Input: part model. Units: mm. Frame: model coordinates. A direction names the side the tool comes from. Coordinates: 2 decimals unless noted, no trailing zeros. Loops run counter-clockwise (first coordinate to the right, second up) from the corner with the lowest first, then second, coordinate; pieces in that order, holes last. Notation, with made-up numbers: (48.25, 72) - (74.25, 72) arc R19 ccw to (74.25, 85) - close; hole circle Ø2 at (-36.75, 76). An arc over 180 degrees is marked (long way). Write item = value, one per line. Start each with the question number.
from build123d import *

# Parameters (mm, degrees)
BOSS_EXTRUDE1_DEPTH   = 4.064
BOSS_EXTRUDE1_2_DEPTH = 4.064
SKETCH1_3_W           = 60.96
SKETCH1_3_H           = 9.652
SKETCH1_3_H_2         = 1.778
BOSS_EXTRUDE2_DEPTH   = 1.524
SKETCH1_6_W           = 60.96
SKETCH1_6_H           = 1.778
BOSS_EXTRUDE3_DEPTH   = 24.13
BOSS_EXTRUDE4_DEPTH   = 38.1
BOSS_EXTRUDE7_DEPTH   = 60.96
BOSS_EXTRUDE8_DEPTH   = 60.96
CUT_EXTRUDE2_START    = -5.08
CUT_EXTRUDE2_DEPTH    = 50.8
SKETCH6_R             = 2.54
CUT_EXTRUDE3_DEPTH    = 89.450736232
BOSS_EXTRUDE9_START   = -27.94
BOSS_EXTRUDE9_DEPTH   = 5.08
BOSS_EXTRUDE10_REACH  = 83.27
CUT_EXTRUDE4_START    = -1.778
CUT_EXTRUDE4_DEPTH    = 57.404


with BuildPart() as part:
    # Sketch1 → Boss-Extrude1 (new body)
    with BuildSketch(Plane(origin=(0, 0, 0), x_dir=(0, 0, -1), z_dir=(1, 0, 0))):
        Polygon((7.62, 0), (0, 0), (0, -11.43), (7.62, -11.43), (7.62, -1.778), align=None)
    extrude(amount=BOSS_EXTRUDE1_DEPTH)



with BuildPart() as body_2:
    # Sketch1 → Boss-Extrude1 2 (new body)
    with BuildSketch(Plane(origin=(0, 0, 0), x_dir=(0, 0, -1), z_dir=(1, 0, 0))):
        Polygon((76.2, 0), (68.58, 0), (68.58, -1.778), (68.58, -11.43), (76.2, -11.43), align=None)
    extrude(amount=BOSS_EXTRUDE1_2_DEPTH)


with BuildPart() as part_1:
    add(part.part)

    add(body_2.part)  # Boss-Extrude2 merges body 2
    # Sketch1<3> → Boss-Extrude2 (add)
    with BuildSketch(Plane(origin=(0, 0, 0), x_dir=(0, 0, -1), z_dir=(1, 0, 0))):
        with Locations((38.1, -6.604)):
            Rectangle(SKETCH1_3_W, SKETCH1_3_H)
        with Locations((38.1, -0.889)):
            Rectangle(SKETCH1_3_W, SKETCH1_3_H_2)
    extrude(amount=BOSS_EXTRUDE2_DEPTH)

    # Sketch1<6> → Boss-Extrude3 (add)
    with BuildSketch(Plane(origin=(0, 0, 0), x_dir=(0, 0, -1), z_dir=(1, 0, 0))):
        with Locations((38.1, -0.889)):
            Rectangle(SKETCH1_6_W, SKETCH1_6_H)
    extrude(amount=-BOSS_EXTRUDE3_DEPTH)

    # Sketch4 → Boss-Extrude4 (add)
    with BuildSketch(Plane.XZ.offset(1.778)):
        Polygon((0, -7.62), (-24.13, -7.62), (-24.13, -68.58), (0, -68.58), (0, -66.802), (-22.352, -66.802), (-22.352, -9.398), (0, -9.398), align=None)
    extrude(amount=-BOSS_EXTRUDE4_DEPTH)

    # Sketch5<4> → Boss-Extrude7 (add)
    with BuildSketch(Plane(origin=(0, 0, -68.58), x_dir=(-1, 0, 0), z_dir=(0, 0, -1))):
        Polygon((1.778, -1.778), (0, -1.778), (0, -3.556), align=None)
    extrude(amount=-BOSS_EXTRUDE7_DEPTH)

    # Sketch5<5> → Boss-Extrude8 (add)
    with BuildSketch(Plane(origin=(0, 0, -68.58), x_dir=(-1, 0, 0), z_dir=(0, 0, -1))):
        Polygon((9.652, -1.778), (5.842, -1.778), (0, -7.62), (0, -11.43), align=None)
    extrude(amount=-BOSS_EXTRUDE8_DEPTH)

    # Sketch5 → Cut-Extrude2 (cut)
    with BuildSketch(Plane(origin=(0, 0, -68.58), x_dir=(-1, 0, 0), z_dir=(0, 0, -1)).offset(CUT_EXTRUDE2_START)):
        Polygon((9.652, -1.778), (5.842, -1.778), (0, -7.62), (0, -11.43), align=None)
    extrude(amount=-CUT_EXTRUDE2_DEPTH, mode=Mode.SUBTRACT)

    # Sketch6 → Cut-Extrude3 (cut, through all)
    with BuildSketch(Plane(origin=(-22.352, 0, 0), x_dir=(0, 0, -1), z_dir=(1, 0, 0))):
        with Locations((23.114, 29.21)):
            Circle(SKETCH6_R)
        with Locations((53.086, 29.21)):
            Circle(SKETCH6_R)
        Polygon((38.1, 20.32), (12.7, 20.32), (12.7, 8.89), (63.5, 8.89), (63.5, 20.32), align=None)
    extrude(amount=-CUT_EXTRUDE3_DEPTH, mode=Mode.SUBTRACT)

    # Sketch5<12> → Boss-Extrude9 (add)
    with BuildSketch(Plane(origin=(0, 0, -68.58), x_dir=(-1, 0, 0), z_dir=(0, 0, -1)).offset(BOSS_EXTRUDE9_START)):
        Polygon((9.652, -1.778), (5.842, -1.778), (0, -7.62), (0, -11.43), align=None)
    extrude(amount=-BOSS_EXTRUDE9_DEPTH)

    # Boss-Extrude10: up to this face of the body (flat: up to its plane)
    boss_extrude10_end = Plane(part_1.part.faces().sort_by_distance((-11.79395977, 16.525022989, -68.58))[0])
    # Sketch9 → Boss-Extrude10 (add, up to the picked face)
    with BuildSketch(Plane.XY.offset(-7.62), mode=Mode.PRIVATE) as boss_extrude10_sk1:
        Polygon((0, 27.94), (0, 30.988), (4.572, 30.988), (4.572, 33.02), (7.140253406, 30.988), (7.140253406, 27.94), align=None)
    boss_extrude10_tool1 = split(extrude(boss_extrude10_sk1.sketch, amount=-BOSS_EXTRUDE10_REACH, mode=Mode.PRIVATE), bisect_by=boss_extrude10_end, keep=Keep.BOTH, mode=Mode.PRIVATE)
    add(boss_extrude10_tool1.solids().sort_by(Axis((3.769039, 29.699674, -7.62), (0, 0, -1)))[0])

    # Sketch9<2> → Cut-Extrude4 (cut)
    with BuildSketch(Plane.XY.offset(-7.62).offset(CUT_EXTRUDE4_START)):
        Polygon((0, 27.94), (0, 30.988), (4.572, 30.988), (4.572, 33.02), (7.140253406, 30.988), (7.140253406, 27.94), align=None)
    extrude(amount=-CUT_EXTRUDE4_DEPTH, mode=Mode.SUBTRACT)


solid = part_1.part
Item 1: Pin query (flat end, axial travel): pin 1 (1 mm diameter, centred on x = -4.5, y = 26.5, fed in from +Z); pin 2 (13 mm diameter, centred on x = -9.5, z = -42, fed in from +Y); pin 3 (2 mm diameter, centred on y = 19.5, z = -9, fed in from +X). Return the tip coordinate at first contact, or that it passes through.
Item 2: Pull-direction query (Z, two-part tool) for faces 1 (the flat face through (-12, 18, -7.62)), 2 (the flat face through (-12, 18, -68.58)), 3 (the flat face through (-24.13, 22, -38)), 4 (the flat face through (-23, 15, -12.7)); classes: pulls with the +Z half, pulls with the -Z half, needs draft (parallel to the pull), parting line crosses it, or undercut.
Item 3: Cut plane C-C on y = -5. Return loops of the section in (x, z), plus the area to 3 significant figures.
Item 4: Ray query, line 1 (Z direction, x = -23, y = 29); line 2 (Z direction, x = -2.5, y = -5.5); line 3 (Z direction, x = -21, y = 2.5). Return the intervals inside material, ascending.
Item 5: Access query for faces 5 (the flat face through (0, 34, -68)), 6 (the flat face through (4, 27.94, -68)), 7 (the flat face through (-2.96, -4.66, -38.14)), 8 (the flat face through (-11, 18, -9.398)). Directions: +Z, -Z, +X, -X, +Y, -Y. A direction counts if a zero-diameter tool reaches every point of the face in a straight line with its end or side. Return the directions, or none.
Item 6: Cut plane A-A on y = 29.21. Return loops of the section in (x, z).
Item 7: Cut plane D-D on x = -21. Return loops of the section in (y, z), plus the area to 3 significant figures.
Item 8: Cut plane B-B on y = 12.5. Return loops of the section in (x, z), plus the area to 3 significant figures.
Recorded:
q1.pin_1 = -7.62
q1.pin_2 = 0
q1.pin_3 = 0
q2.face_1 = pulls with the +Z half
q2.face_2 = pulls with the -Z half
q2.face_3 = needs draft
q2.face_4 = undercut
q3.outline = (-6.43, -68.58) - (-2.62, -68.58) - (-2.62, -63.5) - (-6.43, -63.5) - close; (-6.43, -40.64) - (-2.62, -40.64) - (-2.62, -35.56) - (-6.43, -35.56) - close; (-6.43, -12.7) - (-2.62, -12.7) - (-2.62, -7.62) - (-6.43, -7.62) - close; (0, -76.2) - (4.06, -76.2) - (4.06, -68.58) - (1.52, -68.58) - (1.52, -7.62) - (4.06, -7.62) - (4.06, 0) - (0, 0) - close
q3.area = 213 mm²
q4.line_1 = -68.58 to -55.62, -50.55 to -25.65, -20.58 to -7.62
q4.line_2 = -68.58 to -63.5, -40.64 to -35.56, -12.7 to -7.62
q4.line_3 = -68.58 to -66.8, -9.4 to -7.62
q5.face_5 = +Z, -Z, +Y
q5.face_6 = +Z, -Z, +X
q5.face_7 = +Z, -Z
q5.face_8 = +X, +Y
q6.outline = (-24.13, -68.58) - (7.14, -68.58) - (7.14, -66.8) - (-22.35, -66.8) - (-22.35, -55.63) - (-24.13, -55.63) - close; (-24.13, -50.55) - (-22.35, -50.55) - (-22.35, -25.65) - (-24.13, -25.65) - close; (-24.13, -20.57) - (-22.35, -20.57) - (-22.35, -9.4) - (7.14, -9.4) - (7.14, -7.62) - (-24.13, -7.62) - close
q7.outline = (-1.78, -68.58) - (36.32, -68.58) - (36.32, -66.8) - (0, -66.8) - (0, -9.4) - (36.32, -9.4) - (36.32, -7.62) - (-1.78, -7.62) - close
q7.area = 238 mm²
q8.outline = (-24.13, -68.58) - (0, -68.58) - (0, -66.8) - (-22.35, -66.8) - (-22.35, -63.5) - (-24.13, -63.5) - close; (-24.13, -12.7) - (-22.35, -12.7) - (-22.35, -9.4) - (0, -9.4) - (0, -7.62) - (-24.13, -7.62) - close
q8.area = 97.5 mm²
